Here's how the part is built. I have some questions about the finished solid (model axes, mm). Face numbers are marked on the shaded views. A direction names the side the tool comes from. Give positions to 0.01 mm unless a question says otherwise; leave off trailing zeros. Write each loop counter-clockwise with the first axis right and the second up, starting at its lowest first coordinate (ties: lowest second). Pieces come first, ordered by that corner, then holes. Notation, with made-up numbers: M 34,-21.75 L 42,-21.75 A25 cw 42,-2.75 Z; hole C -20,55.5 d4. An arc over 180 degrees is marked long. Answer as CSV lines item,"result". Start each with the question number.
Q1. If I drill on line 1 along X through (y, z) = (-15.5, 33.5); line 2 along Z through (x, y) = (-17.5, -14); line 3 along X through (y, z) = (-5, 23), over which ranges is the centre line in solid material (lowest first)?
Q2. Suppose I cut it at A-A (x = -11). Write out the boundary of the cut face in (y, z), then the cut area to 3 significant figures.
Q3. On a 3-axis mill with a long thin cutter (end or side, diameter ignored), from which of +Z, -Z, +X, -X, +Y, -Y can I reach the whole of each face in a straight line? I mean the marked faces 4, 5 and 6. Say none if no direction works.
Q4. Thinking about a two-plate mould opening in X: for the marked faces 1, 2 and 3, which applies, +X half, -X half, draft (parallel to the pull), parting line (faces both ways), or undercut?
Q5. Suppose I cut it at C-C (y = -7.5). Write out the boundary of the cut face in (x, z), then the cut area to 3 significant figures.
Q6. For pin 1 (1.5 mm diameter, centred on y = 7.5, z = 7, fed in from -X); pin 2 (6 mm diameter, centred on x = 7.5, z = 12, fed in from -Y); pin 3 (4.5 mm diameter, centred on x = 12.8, y = 0.34, fed in from +Z) (1 decimal); pin 4 (10 mm diameter, centred on x = -4, z = 14.5, fed in from +Y), each with a flat end and sliding along its axis, tell me the tip position at first contact or that it passes through.
Autodesk Inventor part; units mm, degrees
ref_plane "Work Plane2" through (-93.6315, -146.1207, 0) normal (0, 0, 1) x (1, 0, 0)
ref_plane "YZ Plane" through (0, 0, 0) normal (1, 0, 0) x (0, 1, 0)
ref_plane "XZ Plane" through (0, 0, 0) normal (0, 1, 0) x (-1, 0, 0)
ref_plane "Work Plane1" through (1.0078, -6.2592, 14.7955) normal (0, 0, -1) x (0.9872698, 0.1590547, 0)
sketch "Sketch1" plane through (1.0078, -6.2592, 14.7955) normal (0, 0, -1) x (0.9872698, 0.1590547, 0)
  circle A0 centre (12.6864, -4.6373) radius 2.9337
  circle A1 centre (-12.7136, -4.6337) radius 2.9337
  line L0 (25.2845, 14.4163) -> (-25.5155, 14.4163)
  line L1 (-25.5155, 14.4163) -> (-25.5155, -23.6837)
  line L2 (-25.5155, -23.6837) -> (25.2845, -23.6837)
  line L3 (25.2845, -23.6837) -> (25.2845, 14.4163)
  point P0 (0.0006, -6.3398)
  dimension "d0" = 50.8
  dimension "d1" = 38.1
  dimension "d2" = 19.05
  dimension "d3" = 12.8018
ref_plane "Work Plane2" through (-93.6315, -146.1207, 0) normal (0, 0, 1) x (1, 0, 0)
extrude "Extrusion1" add sketch "Sketch1" along normal up to surface (14.7955 mm away)
sketch "Sketch2" plane through (1.0078, -6.2592, 14.7955) normal (0, 0, 1) x (0.9872698, 0.1590547, 0)
  line L0 (6.35, -58.321) -> (6.35, 48.9196)
  line L1 (-6.35, 49.2476) -> (-6.35, -58.321)
  circle A0 centre (-12.7136, 4.6337) radius 2.9337
  circle A1 centre (12.6864, 4.6373) radius 2.9337
  line L2 (25.2845, -14.4163) -> (-25.5155, -14.4163)
  line L3 (25.2845, 23.6837) -> (25.2845, -14.4163)
  line L4 (-25.5155, 23.6837) -> (25.2845, 23.6837)
  line L5 (-25.5155, -14.4163) -> (-25.5155, 23.6837)
  line L6 (25.2845, -14.4163) -> (-25.5155, -14.4163)
  line L7 (25.2845, -14.4163) -> (7.62, -14.4163)
  line L8 (7.62, -14.4163) -> (7.62, 23.6837)
  line L9 (7.62, 23.6837) -> (25.2845, 23.6837)
  line L10 (25.2845, 23.6837) -> (25.2845, -14.4163)
  line L11 (-25.5155, -14.4163) -> (-25.5155, 23.6837)
  line L12 (-25.5155, -14.4163) -> (-7.62, -14.4163)
  line L13 (-7.62, -14.4163) -> (-7.62, 23.6837)
  line L14 (-7.62, 23.6837) -> (-25.5155, 23.6837)
  line L15 (-25.5155, 23.6837) -> (-25.5155, -14.4163)
  point P0 (0.0006, 6.3398)
  dimension "d6" = 1.27
  dimension "d7" = 1.27
extrude "Extrusion2" add sketch "Sketch2" along normal blind 25.4 contours L8 L4 L3 L2 | L2 L5 L4 L13
shell "Shell1" thickness 3.81 removed faces 0
properties part number "wrench holder"
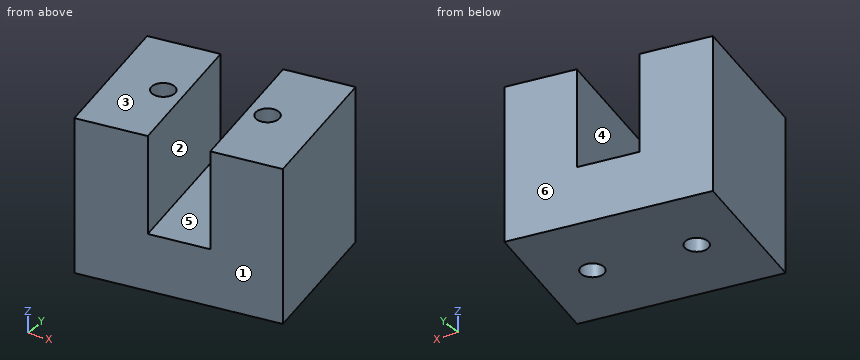
Resolved:
1,line 1,"-23.35 to -19.49, -9.08 to -5.22, 10.21 to 28.11"
1,line 2,"0 to 3.81, 36.39 to 40.2"
1,line 3,"-25.04 to -21.18, -18.9 to -14.91, -9.65 to -6.91, 8.52 to 16.92, 22.56 to 26.42"
2,outline,"M -22.8,0 L -6.35,0 L -6.35,40.2 L -22.8,40.2 Z; M -1.07,0 L 15.8,0 L 15.8,40.2 L -1.07,40.2 Z; hole M -18.94,3.81 L -10.33,3.81 L -10.33,36.39 L -18.94,36.39 Z; hole M 2.91,3.81 L 11.94,3.81 L 11.94,10.99 L 2.91,10.99 Z"
2,area,"994 mm^2"
3,face 4,"+Z, -Y"
3,face 5,"+Z"
3,face 6,"+Z, -Z, -X, +Y"
4,face 1,"+X half"
4,face 2,"undercut"
4,face 3,"draft"
5,outline,"M -24.64,0 L 26.82,0 L 26.82,40.2 L 8.93,40.2 L 8.93,14.8 L -6.51,14.8 L -6.51,40.2 L -24.64,40.2 Z; hole M -20.78,3.81 L -17.86,3.81 L -17.86,36.39 L -20.78,36.39 Z; hole M -6.71,3.81 L 22.96,3.81 L 22.96,36.39 L 12.79,36.39 L 12.79,10.99 L -6.71,10.99 Z"
5,area,"1,110 mm^2"
6,pin 1,"x = -27.17"
6,pin 2,"y = -20.3"
6,pin 3,"through"
6,pin 4,"y = 17.73"
